Check sheet for the modelled part. Datum: model origin and axes. Units: mm. A direction names the side the tool comes from. Round coordinates to 2 decimals unless told otherwise and drop trailing zeros. Write each loop counter-clockwise with the first axis right and the second up, starting at its lowest first coordinate (ties: lowest second). Pieces come first, ordered by that corner, then holes. Notation, with made-up numbers: M -40,56.5 L 9,56.5 A34 cw 9,89.5 Z; hole C 63,64 d1. An arc over 180 degrees is marked long. Answer in a Markdown table with one row per item.
```python
from build123d import *

# Parameters (mm, degrees)
BOSS_EXTRUDE1_DEPTH = 4
CUT_EXTRUDE1_DEPTH  = 4
SKETCH3_R           = 2
SKETCH3_R_2         = 1.5
CUT_EXTRUDE2_DEPTH  = 10
SKETCH4_R           = 1.5
CUT_EXTRUDE3_DEPTH  = 10


with BuildPart() as part:
    # Sketch1 → Boss-Extrude1 (new body)
    with BuildSketch(Plane.XY):
        with BuildLine():
            Line((-95, -115), (-95, -195))
            ThreePointArc((-95, -195), (-93.535533906, -198.535533906), (-90, -200))
            Line((-90, -200), (90, -200))
            ThreePointArc((90, -200), (93.535533906, -198.535533906), (95, -195))
            Line((95, -195), (95, -115))
            ThreePointArc((95, -115), (93.535533906, -111.464466094), (90, -110))
            Line((90, -110), (60, -110))
            ThreePointArc((60, -110), (56.464466094, -108.535533906), (55, -105))
            Line((55, -105), (55, -45))
            ThreePointArc((55, -45), (56.464466094, -41.464466094), (60, -40))
            Line((60, -40), (90, -40))
            ThreePointArc((90, -40), (93.535533906, -38.535533906), (95, -35))
            Line((95, -35), (95, -5))
            ThreePointArc((95, -5), (93.535533906, -1.464466094), (90, 0))
            Line((90, 0), (-90, 0))
            ThreePointArc((-90, 0), (-93.535533906, -1.464466094), (-95, -5))
            Line((-95, -5), (-95, -35))
            ThreePointArc((-95, -35), (-93.535533906, -38.535533906), (-90, -40))
            Line((-90, -40), (-60, -40))
            ThreePointArc((-60, -40), (-56.464466094, -41.464466094), (-55, -45))
            Line((-55, -45), (-55, -105))
            ThreePointArc((-55, -105), (-56.464466094, -108.535533906), (-60, -110))
            Line((-60, -110), (-90, -110))
            ThreePointArc((-90, -110), (-93.535533906, -111.464466094), (-95, -115))
        make_face()
    extrude(amount=BOSS_EXTRUDE1_DEPTH)

    # Sketch2 → Cut-Extrude1 (cut)
    with BuildSketch(Plane.XY.offset(4)):
        with BuildLine():
            Line((-35, -120), (35, -120))
            ThreePointArc((35, -120), (38.535533906, -121.464466094), (40, -125))
            Line((40, -125), (40, -175))
            ThreePointArc((40, -175), (38.535533906, -178.535533906), (35, -180))
            Line((35, -180), (-35, -180))
            ThreePointArc((-35, -180), (-38.535533906, -178.535533906), (-40, -175))
            Line((-40, -175), (-40, -125))
            ThreePointArc((-40, -125), (-38.535533906, -121.464466094), (-35, -120))
        make_face()
    extrude(amount=-CUT_EXTRUDE1_DEPTH, mode=Mode.SUBTRACT)

    # Sketch3 → Cut-Extrude2 (cut)
    with BuildSketch(Plane.XY.offset(4)):
        with Locations((-85, -15)):
            Circle(SKETCH3_R)
        with Locations((-85, -185)):
            Circle(SKETCH3_R)
        with Locations((85, -185)):
            Circle(SKETCH3_R)
        with Locations((85, -15)):
            Circle(SKETCH3_R)
        with Locations((-27, -11)):
            Circle(SKETCH3_R_2)
        with Locations((27, -11)):
            Circle(SKETCH3_R_2)
        with BuildLine():
            Line((-4.5, -7.5), (4.5, -7.5))
            ThreePointArc((4.5, -7.5), (5.914213562, -8.085786438), (6.5, -9.5))
            Line((6.5, -9.5), (6.5, -11.5))
            ThreePointArc((6.5, -11.5), (5.914213562, -12.914213562), (4.5, -13.5))
            Line((4.5, -13.5), (-4.5, -13.5))
            ThreePointArc((-4.5, -13.5), (-5.914213562, -12.914213562), (-6.5, -11.5))
            Line((-6.5, -11.5), (-6.5, -9.5))
            ThreePointArc((-6.5, -9.5), (-5.914213562, -8.085786438), (-4.5, -7.5))
        make_face()
    extrude(amount=-CUT_EXTRUDE2_DEPTH, mode=Mode.SUBTRACT)

    # Sketch4 → Cut-Extrude3 (cut)
    with BuildSketch(Plane.XY.offset(4)):
        with Locations((-71.25, -25)):
            Circle(SKETCH4_R)
        with Locations((-71.25, -75)):
            Circle(SKETCH4_R)
        with Locations((-71.25, -175)):
            Circle(SKETCH4_R)
        with Locations((-71.25, -125)):
            Circle(SKETCH4_R)
        with Locations((-23.75, -125)):
            Circle(SKETCH4_R)
        with Locations((-23.75, -175)):
            Circle(SKETCH4_R)
        with Locations((-23.75, -75)):
            Circle(SKETCH4_R)
        with Locations((-23.75, -25)):
            Circle(SKETCH4_R)
        with Locations((23.75, -25)):
            Circle(SKETCH4_R)
        with Locations((23.75, -75)):
            Circle(SKETCH4_R)
        with Locations((23.75, -175)):
            Circle(SKETCH4_R)
        with Locations((23.75, -125)):
            Circle(SKETCH4_R)
        with Locations((71.25, -125)):
            Circle(SKETCH4_R)
        with Locations((71.25, -175)):
            Circle(SKETCH4_R)
        with Locations((71.25, -75)):
            Circle(SKETCH4_R)
        with Locations((71.25, -25)):
            Circle(SKETCH4_R)
    extrude(amount=-CUT_EXTRUDE3_DEPTH, mode=Mode.SUBTRACT)


solid = part.part
```
1. Section check D-D, the plane y = -93. Record the cut outline in (x, z).
Found:
| item | result |
|---|---|
| outline | M -55,0 L 55,0 L 55,4 L -55,4 Z |
2. Section check C-C, the plane z = 2.75. Count the separate pieces of the cut face and the enclosed holes in it, and give its area (3 significant figures).
Found:
| item | result |
|---|---|
| separate pieces | 1 |
| enclosed holes | 18 |
| area | 27,400 mm2 |
3. Draft check along Y on faces 6 (the face through (94, -2, 2)), 7 (the face through (-38, -179, 2)), 8 (the face through (-1, -99, 4)). Enter one of: +Y half, -Y half, draft (parallel to the pull), parting line (faces both ways), or undercut.
Found:
| item | result |
|---|---|
| face 6 | +Y half |
| face 7 | undercut |
| face 8 | draft |
4. Access from +Z, -Z, +X, -X, +Y, -Y to the whole of each face (thin tool, end or side, straight path). Record for faces 1 (the face through (38, -121, 2)), 2 (the face through (93, -199, 2)), 3 (the face through (-56, -108, 2)), 4 (the face through (-94, -198, 2)), 5 (the face through (94, -112, 2)).
Found:
| item | result |
|---|---|
| face 1 | +Z, -Z |
| face 2 | +Z, -Z, +X, -Y |
| face 3 | +Z, -Z, -X |
| face 4 | +Z, -Z, -X, -Y |
| face 5 | +Z, -Z, +X |
5. Section check A-A, the plane x = -64. Record the cut outline in (y, z).
Found:
| item | result |
|---|---|
| outline | M -200,0 L -110,0 L -110,4 L -200,4 Z; M -40,0 L 0,0 L 0,4 L -40,4 Z |
6. Go/stop test with flat-tipped pins: pin 1 (2.5 mm diameter, centred on x = -27, y = -11, fed in from +Z); pin 2 (2 mm diameter, centred on y = -74.5, z = 2, fed in from +X). Record where each tip stops, or that it passes through.
Found:
| item | result |
|---|---|
| pin 1 | passes through |
| pin 2 | stops at x = 55 |
7. Section check B-B, the plane y = -157. Record the cut outline in (x, z).
Found:
| item | result |
|---|---|
| outline | M -95,0 L -40,0 L -40,4 L -95,4 Z; M 40,0 L 95,0 L 95,4 L 40,4 Z |
8. Scan lines: L1, parallel to Y at x = 23.75, z = 1.6; L2, parallel to X at y = -75, z = 2.1; L3, parallel to Y at x = 3.5, z = 3.1. Record each from-to range of solid material in increasing order.
Found:
| item | result |
|---|---|
| L1 | y = -200 to -180, -120 to -76.5, -73.5 to -26.5, -23.5 to 0 |
| L2 | x = -55 to -25.25, -22.25 to 22.25, 25.25 to 55 |
| L3 | y = -200 to -180, -120 to -13.5, -7.5 to 0 |
